```python
from build123d import *

# Parameters (mm, degrees)
SKETCH_1_W          = 30
SKETCH_1_H          = 55
EXTRUDE_1_DEPTH     = 40
SKETCH_4_W          = 30
SKETCH_4_H          = 20
CUT_EXTRUDE_1_DEPTH = 58.063561053
SKETCH_5_W          = 15
SKETCH_5_H          = 20
EXTRUDE_3_DEPTH     = 60
SKETCH_6_W          = 40
SKETCH_6_H          = 30
EXTRUDE_4_DEPTH     = 55
SKETCH_7_W          = 25
SKETCH_7_H          = 12
CUT_EXTRUDE_2_DEPTH = 116.352719951


with BuildPart() as part:
    # Эскиз1 → Бобышка-Вытянуть1 (new body)
    with BuildSketch(Plane.XY):
        Rectangle(SKETCH_1_W, SKETCH_1_H)
    extrude(amount=EXTRUDE_1_DEPTH)

    # Эскиз4 → Вырез-Вытянуть1 (cut, through all)
    with BuildSketch(Plane(origin=(15, 0, 0), x_dir=(0, 0, -1), z_dir=(1, 0, 0))):
        with Locations((-20, 7.5)):
            Rectangle(SKETCH_4_W, SKETCH_4_H)
    extrude(amount=-CUT_EXTRUDE_1_DEPTH, mode=Mode.SUBTRACT)

    # Эскиз5 → Бобышка-Вытянуть3 (add)
    with BuildSketch(Plane(origin=(0, 0, 0), x_dir=(-1, 0, 0), z_dir=(0, 0, -1))):
        with Locations((-7.5, -17.5)):
            Rectangle(SKETCH_5_W, SKETCH_5_H)
    extrude(amount=EXTRUDE_3_DEPTH)

    # Эскиз6 → Бобышка-Вытянуть4 (add)
    with BuildSketch(Plane.XZ.offset(27.5)):
        with Locations((20, -45)):
            Rectangle(SKETCH_6_W, SKETCH_6_H)
    extrude(amount=EXTRUDE_4_DEPTH)

    # Эскиз7 → Вырез-Вытянуть2 (cut, through all)
    with BuildSketch(Plane.XY.offset(-30)):
        with Locations((20, -76.5)):
            Rectangle(SKETCH_7_W, SKETCH_7_H)
    extrude(amount=-CUT_EXTRUDE_2_DEPTH, mode=Mode.SUBTRACT)


solid = part.part
```
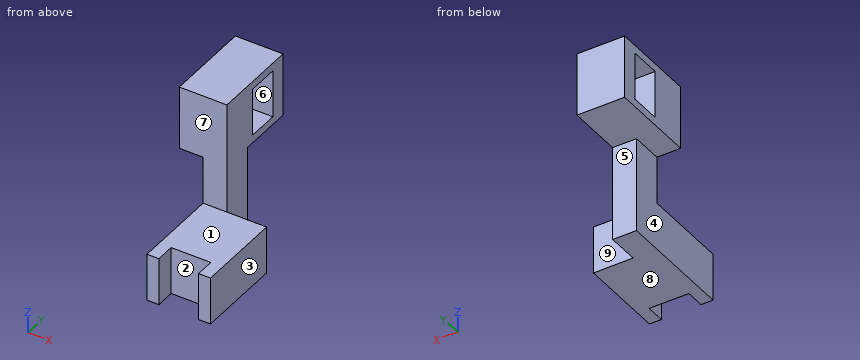
Input: part model. Units: mm. Frame: model coordinates. Face numbers are marked on the shaded views. A direction names the side the tool comes from. Coordinates: 2 decimals unless noted, no trailing zeros. Loops run counter-clockwise (first coordinate to the right, second up) from the corner with the lowest first, then second, coordinate; pieces in that order, holes last. Notation, with made-up numbers: (-34.5, 9) -> (1.5, 9) arc R19 cw to (1.5, 32) -> close; hole circle Ø6 at (20, -2.5). An arc over 180 degrees is marked (long way). Use a Markdown table: item, result.
1) Access query for the marked faces 5, 6, 7, 8 and 9. Directions: +Z, -Z, +X, -X, +Y, -Y. A direction counts if a zero-diameter tool reaches every point of the face in a straight line with its end or side. Return the directions, or none.
Results found:
| item | result |
|---|---|
| face 5 | -Z, +X, -X, +Y |
| face 6 | +X, -X |
| face 7 | +Z, +X, -X, -Y |
| face 8 | -Z, +X, -X, +Y, -Y |
| face 9 | +Z, -Z, +X, +Y |
2) Cut plane A-A (y = -75). Return the cut outline in (x, z).
Results found:
| item | result |
|---|---|
| outline | (0, -60) -> (7.5, -60) -> (7.5, -30) -> (0, -30) -> close; (32.5, -60) -> (40, -60) -> (40, -30) -> (32.5, -30) -> close |
3) Pull-direction query (X, two-part tool) for the marked faces 1, 2, 3 and 4; classes: released by +X, released by -X, zero draft, split by the parting line, or undercut.
Results found:
| item | result |
|---|---|
| face 1 | zero draft |
| face 2 | undercut |
| face 3 | released by +X |
| face 4 | released by -X |
4) Cut plane B-B (z = 15). Return the cut outline in (x, y).
Results found:
| item | result |
|---|---|
| outline | (-15, -27.5) -> (15, -27.5) -> (15, -2.5) -> (-15, -2.5) -> close; (-15, 17.5) -> (15, 17.5) -> (15, 27.5) -> (-15, 27.5) -> close |
5) Contact query for flat-ended pins moving along their axis: pin 1 (1.5 mm diameter, centred on x = 7, y = 14.5, fed in from -Z); pin 2 (8 mm diameter, centred on x = 8.5, z = -4, fed in from -Y); pin 3 (13 mm diameter, centred on y = -78, z = -39, fed in from -X). Output: stop coordinate, or through.
Results found:
| item | result |
|---|---|
| pin 1 | stops at z = 0 |
| pin 2 | stops at y = -27.5 |
| pin 3 | stops at x = 0 |
6) Cut plane C-C (x = -6). Return the cut outline in (y, z), then the cut area to 3 significant figures.
Results found:
| item | result |
|---|---|
| outline | (-27.5, 0) -> (27.5, 0) -> (27.5, 40) -> (-27.5, 40) -> close; hole (-2.5, 5) -> (17.5, 5) -> (17.5, 35) -> (-2.5, 35) -> close |
| area | 1,600 mm2 |
7) Cut plane D-D (z = -37.5). Return the cut outline in (x, y), then the cut area to 3 significant figures.
Results found:
| item | result |
|---|---|
| outline | (0, -82.5) -> (7.5, -82.5) -> (7.5, -70.5) -> (32.5, -70.5) -> (32.5, -82.5) -> (40, -82.5) -> (40, -27.5) -> (15, -27.5) -> (15, -7.5) -> (0, -7.5) -> close |
| area | 2,200 mm2 |
8) Material intervals for line 1 along Z through (x, y) = (-6, 5.5); line 2 along Y through (x, z) = (7.5, 13); line 3 along X through (y, z) = (-71.5, -32), sorted ascending. Write a range as from..to.
Results found:
| item | result |
|---|---|
| line 1 | z = 0..5, 35..40 |
| line 2 | y = -27.5..-2.5, 17.5..27.5 |
| line 3 | x = 0..7.5, 32.5..40 |
